CAD build for the part. Positions are in the model's coordinates, mm. Face numbers are marked on the shaded views. Coordinates: 2 decimals unless noted, no trailing zeros. Write each loop counter-clockwise with the first axis right and the second up, starting at its lowest first coordinate (ties: lowest second). Pieces come first, ordered by that corner, then holes. Notation, with made-up numbers: M -12,-20 L -5,-20 A13 cw -5,1 Z; hole C -12.75,-28 d2. An arc over 180 degrees is marked long. Answer as CSV lines item,"result". Start each with the question number.
```python
from build123d import *

# Parameters (mm, degrees)
BOSS_EXTRUDE1_DEPTH = 6
CUT_EXTRUDE1_DEPTH  = 5


with BuildPart() as part:
    # Sketch1 → Boss-Extrude1 (new body)
    with BuildSketch(Plane(origin=(0, 0, 0), x_dir=(1, 0, 0), z_dir=(0, 1, 0))):
        with BuildLine():
            Line((10, 0), (267, 0))
            ThreePointArc((267, 0), (274.071067812, 2.928932188), (277, 10))
            Line((277, 10), (277, 276))
            ThreePointArc((277, 276), (274.071067812, 283.071067812), (267, 286))
            Line((267, 286), (10, 286))
            ThreePointArc((10, 286), (2.928932188, 283.071067812), (0, 276))
            Line((0, 276), (0, 10))
            ThreePointArc((0, 10), (2.928932188, 2.928932188), (10, 0))
        make_face()
    extrude(amount=BOSS_EXTRUDE1_DEPTH)

    # Sketch2 → Cut-Extrude1 (cut)
    with BuildSketch(Plane(origin=(0, 6, 0), x_dir=(1, 0, 0), z_dir=(0, 1, 0))):
        with BuildLine():
            Line((12, 12), (22.5, 12))
            Line((22.5, 12), (22.5, 20.5))
            ThreePointArc((22.5, 20.5), (26.5, 24.5), (30.5, 20.5))
            Line((30.5, 20.5), (30.5, 12))
            Line((30.5, 12), (66.5, 12))
            Line((66.5, 12), (66.5, 20.5))
            ThreePointArc((66.5, 20.5), (70.5, 24.5), (74.5, 20.5))
            Line((74.5, 20.5), (74.5, 12))
            Line((74.5, 12), (85.5, 12))
            Line((85.5, 12), (85.5, 92))
            Line((85.5, 92), (83.159502005, 102.5))
            Line((83.159502005, 102.5), (83.159502005, 124.5))
            Line((83.159502005, 124.5), (72.459502005, 124.5))
            Line((72.459502005, 124.5), (72.459502005, 134.7))
            Line((72.459502005, 134.7), (54.459502005, 134.7))
            Line((54.459502005, 134.7), (54.459502005, 124.5))
            Line((54.459502005, 124.5), (42.659513404, 124.5))
            Line((42.659513404, 124.5), (42.659513404, 134.663480988))
            Line((42.659513404, 134.663480988), (24.659513404, 134.663480988))
            Line((24.659513404, 134.663480988), (24.659513404, 124.463480988))
            ThreePointArc((24.659513404, 124.463480988), (17.228582428, 121.834216678), (14.340497995, 114.5))
            Line((14.340497995, 114.5), (14.340497995, 102.5))
            Line((14.340497995, 102.5), (12, 92))
            Line((12, 92), (12, 12))
        make_face()
        with BuildLine():
            Line((114.659513404, 124.463480988), (114.659513404, 134.663480988))
            Line((114.659513404, 134.663480988), (132.659513404, 134.663480988))
            Line((132.659513404, 134.663480988), (132.659513404, 124.5))
            Line((132.659513404, 124.5), (144.459502005, 124.5))
            Line((144.459502005, 124.5), (144.459502005, 134.7))
            Line((144.459502005, 134.7), (162.459502005, 134.7))
            Line((162.459502005, 134.7), (162.459502005, 124.5))
            Line((162.459502005, 124.5), (173.159502005, 124.5))
            Line((173.159502005, 124.5), (173.159502005, 102.5))
            Line((173.159502005, 102.5), (175.5, 92))
            Line((175.5, 92), (175.5, 12))
            Line((175.5, 12), (164.5, 12))
            Line((164.5, 12), (164.5, 20.5))
            ThreePointArc((164.5, 20.5), (160.5, 24.5), (156.5, 20.5))
            Line((156.5, 20.5), (156.5, 12))
            Line((156.5, 12), (120.5, 12))
            Line((120.5, 12), (120.5, 20.5))
            ThreePointArc((120.5, 20.5), (116.5, 24.5), (112.5, 20.5))
            Line((112.5, 20.5), (112.5, 12))
            Line((112.5, 12), (102, 12))
            Line((102, 12), (102, 92))
            Line((102, 92), (104.340497995, 102.5))
            Line((104.340497995, 102.5), (104.340497995, 114.5))
            ThreePointArc((104.340497995, 114.5), (107.228582428, 121.834216678), (114.659513404, 124.463480988))
        make_face()
        with BuildLine():
            Line((204.659513404, 124.463480988), (204.659513404, 134.663480988))
            Line((204.659513404, 134.663480988), (222.659513404, 134.663480988))
            Line((222.659513404, 134.663480988), (222.659513404, 124.5))
            Line((222.659513404, 124.5), (234.459502005, 124.5))
            Line((234.459502005, 124.5), (234.459502005, 134.7))
            Line((234.459502005, 134.7), (252.459502005, 134.7))
            Line((252.459502005, 134.7), (252.459502005, 124.5))
            Line((252.459502005, 124.5), (263.159502005, 124.5))
            Line((263.159502005, 124.5), (263.159502005, 102.5))
            Line((263.159502005, 102.5), (265.5, 92))
            Line((265.5, 92), (265.5, 12))
            Line((265.5, 12), (254.5, 12))
            Line((254.5, 12), (254.5, 20.5))
            ThreePointArc((254.5, 20.5), (250.5, 24.5), (246.5, 20.5))
            Line((246.5, 20.5), (246.5, 12))
            Line((246.5, 12), (210.5, 12))
            Line((210.5, 12), (210.5, 20.5))
            ThreePointArc((210.5, 20.5), (206.5, 24.5), (202.5, 20.5))
            Line((202.5, 20.5), (202.5, 12))
            Line((202.5, 12), (192, 12))
            Line((192, 12), (192, 92))
            Line((192, 92), (194.340497995, 102.5))
            Line((194.340497995, 102.5), (194.340497995, 114.5))
            ThreePointArc((194.340497995, 114.5), (197.228582428, 121.834216678), (204.659513404, 124.463480988))
        make_face()
        with BuildLine():
            Line((114.659513404, 264.463480988), (114.659513404, 274.663480988))
            Line((114.659513404, 274.663480988), (132.659513404, 274.663480988))
            Line((132.659513404, 274.663480988), (132.659513404, 264.5))
            Line((132.659513404, 264.5), (144.459502005, 264.5))
            Line((144.459502005, 264.5), (144.459502005, 274.7))
            Line((144.459502005, 274.7), (162.459502005, 274.7))
            Line((162.459502005, 274.7), (162.459502005, 264.5))
            Line((162.459502005, 264.5), (173.159502005, 264.5))
            Line((173.159502005, 264.5), (173.159502005, 242.5))
            Line((173.159502005, 242.5), (175.5, 232))
            Line((175.5, 232), (175.5, 152))
            Line((175.5, 152), (164.5, 152))
            Line((164.5, 152), (164.5, 160.5))
            ThreePointArc((164.5, 160.5), (160.5, 164.5), (156.5, 160.5))
            Line((156.5, 160.5), (156.5, 152))
            Line((156.5, 152), (120.5, 152))
            Line((120.5, 152), (120.5, 160.5))
            ThreePointArc((120.5, 160.5), (116.5, 164.5), (112.5, 160.5))
            Line((112.5, 160.5), (112.5, 152))
            Line((112.5, 152), (102, 152))
            Line((102, 152), (102, 232))
            Line((102, 232), (104.340497995, 242.5))
            Line((104.340497995, 242.5), (104.340497995, 254.5))
            ThreePointArc((104.340497995, 254.5), (107.228582428, 261.834216678), (114.659513404, 264.463480988))
        make_face()
        with BuildLine():
            Line((204.659513404, 264.463480988), (204.659513404, 274.663480988))
            Line((204.659513404, 274.663480988), (222.659513404, 274.663480988))
            Line((222.659513404, 274.663480988), (222.659513404, 264.5))
            Line((222.659513404, 264.5), (234.459502005, 264.5))
            Line((234.459502005, 264.5), (234.459502005, 274.7))
            Line((234.459502005, 274.7), (252.459502005, 274.7))
            Line((252.459502005, 274.7), (252.459502005, 264.5))
            Line((252.459502005, 264.5), (263.159502005, 264.5))
            Line((263.159502005, 264.5), (263.159502005, 242.5))
            Line((263.159502005, 242.5), (265.5, 232))
            Line((265.5, 232), (265.5, 152))
            Line((265.5, 152), (254.5, 152))
            Line((254.5, 152), (254.5, 160.5))
            ThreePointArc((254.5, 160.5), (250.5, 164.5), (246.5, 160.5))
            Line((246.5, 160.5), (246.5, 152))
            Line((246.5, 152), (210.5, 152))
            Line((210.5, 152), (210.5, 160.5))
            ThreePointArc((210.5, 160.5), (206.5, 164.5), (202.5, 160.5))
            Line((202.5, 160.5), (202.5, 152))
            Line((202.5, 152), (192, 152))
            Line((192, 152), (192, 232))
            Line((192, 232), (194.340497995, 242.5))
            Line((194.340497995, 242.5), (194.340497995, 254.5))
            ThreePointArc((194.340497995, 254.5), (197.228582428, 261.834216678), (204.659513404, 264.463480988))
        make_face()
        with BuildLine():
            Line((24.659513404, 264.463480988), (24.659513404, 274.663480988))
            Line((24.659513404, 274.663480988), (42.659513404, 274.663480988))
            Line((42.659513404, 274.663480988), (42.659513404, 264.5))
            Line((42.659513404, 264.5), (54.459502005, 264.5))
            Line((54.459502005, 264.5), (54.459502005, 274.7))
            Line((54.459502005, 274.7), (72.459502005, 274.7))
            Line((72.459502005, 274.7), (72.459502005, 264.5))
            Line((72.459502005, 264.5), (83.159502005, 264.5))
            Line((83.159502005, 264.5), (83.159502005, 242.5))
            Line((83.159502005, 242.5), (85.5, 232))
            Line((85.5, 232), (85.5, 152))
            Line((85.5, 152), (74.5, 152))
            Line((74.5, 152), (74.5, 160.5))
            ThreePointArc((74.5, 160.5), (70.5, 164.5), (66.5, 160.5))
            Line((66.5, 160.5), (66.5, 152))
            Line((66.5, 152), (30.5, 152))
            Line((30.5, 152), (30.5, 160.5))
            ThreePointArc((30.5, 160.5), (26.5, 164.5), (22.5, 160.5))
            Line((22.5, 160.5), (22.5, 152))
            Line((22.5, 152), (12, 152))
            Line((12, 152), (12, 232))
            Line((12, 232), (14.340497995, 242.5))
            Line((14.340497995, 242.5), (14.340497995, 254.5))
            ThreePointArc((14.340497995, 254.5), (17.228582428, 261.834216678), (24.659513404, 264.463480988))
        make_face()
    extrude(amount=-CUT_EXTRUDE1_DEPTH, mode=Mode.SUBTRACT)


solid = part.part
```
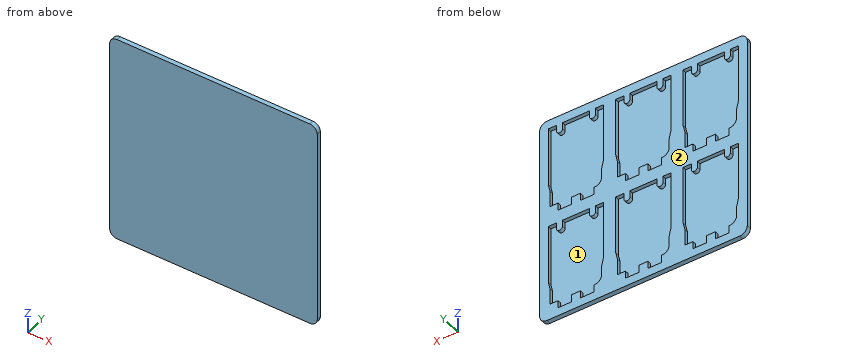
1) Two-plate mould, pull along X, no slides. Class the marked faces 1 and 2: pulls with the +X half, pulls with the -X half, needs draft (parallel to the pull), parting line crosses it, or undercut.
2) Band-saw the part on B-B, the plane x = 226. List the corners of the cut face in (y, z).
3) Band-saw the part on D-D, the plane z = -216.5. List the corners of the cut face in (x, y).
4) Probe L1, parallel to X at y = 2.8, z = -86.5; L2, parallel to Z at x = 75, y = 3.4; L3, parallel to Z at x = 31, y = 3.55. List the from-to ranges inside material, lowest first. Write a range as [from, to].
5) Pin check, flat tips, straight feed: P1, Ø5, axis at x = 222, z = -88, coming from the -Y side; P2, Ø1, axis at x = 107, z = -85.5, coming from the +Y side. Stop position of each tip, or through.
6) Band-saw the part on C-C, the plane y = 3.9. State how many separate pieces and enclosed holes the cut face has, plus the area to 3 significant figures.
7) Band-saw the part on A-A, the plane z = -106. List the corners of the cut face in (x, y).
Result sheet:
1,face 1,"undercut"
1,face 2,"needs draft"
2,outline,"M 0,-286 L 6,-286 L 6,-264.5 L 1,-264.5 L 1,-152 L 6,-152 L 6,-124.5 L 1,-124.5 L 1,-12 L 6,-12 L 6,0 L 0,0 Z"
3,outline,"M 0,0 L 277,0 L 277,6 L 265.5,6 L 265.5,1 L 192,1 L 192,6 L 175.5,6 L 175.5,1 L 102,1 L 102,6 L 85.5,6 L 85.5,1 L 12,1 L 12,6 L 0,6 Z"
4,L1,"x = [0, 12], [85.5, 102], [175.5, 192], [265.5, 277]"
4,L2,"z = [-286, -264.5], [-152, -124.5], [-12, 0]"
4,L3,"z = [-286, -274.66], [-152, -134.66], [-12, 0]"
5,P1,"stops at y = 0"
5,P2,"stops at y = 1"
6,separate pieces,"1"
6,enclosed holes,"6"
6,area,"29,300 mm²"
7,outline,"M 0,0 L 277,0 L 277,6 L 263.16,6 L 263.16,1 L 194.34,1 L 194.34,6 L 173.16,6 L 173.16,1 L 104.34,1 L 104.34,6 L 83.16,6 L 83.16,1 L 14.34,1 L 14.34,6 L 0,6 Z"
